```python
from build123d import *

# Parameters (mm, degrees)
BOSS_EXTRUDE1_DEPTH     = 5
SKETCH2_W               = 30
SKETCH2_H               = 15
BOSS_EXTRUDE2_DEPTH     = 25
CUT_EXTRUDE1_DEPTH      = 44.373378932
SKETCH3_3_R             = 14
SKETCH3_3_R_2           = 13
CUT_EXTRUDE2_DEPTH      = 1
CUT_EXTRUDE3_DEPTH      = 44.373378932
CUT_EXTRUDE3_DEPTH_BACK = 44.373378932
SKETCH3_4_R             = 4
SKETCH3_5_R             = 13
SKETCH3_5_R_2           = 5
CUT_EXTRUDE4_DEPTH      = 3
CUT_EXTRUDE5_START      = 3
SKETCH5_R               = 13
SKETCH5_R_2             = 5
CUT_EXTRUDE5_DEPTH      = 3
CUT_EXTRUDE8_START      = 1
SKETCH5_8_R             = 14
SKETCH5_8_R_2           = 13
CUT_EXTRUDE8_DEPTH      = 1
CUT_EXTRUDE9_START      = 2
SKETCH5_9_R             = 5
SKETCH5_9_R_2           = 4
CUT_EXTRUDE9_DEPTH      = 2
SKETCH6_R               = 2.65
CUT_EXTRUDE10_DEPTH     = 38.91437722


with BuildPart() as part:
    # Sketch1 → Boss-Extrude1 (new body)
    with BuildSketch(Plane(origin=(0, 0, 0), x_dir=(1, 0, 0), z_dir=(0, 1, 0))):
        Polygon((25.5, 7.5), (27.5, 5.5), (27.5, -5.5), (25.5, -7.5), (-25.5, -7.5), (-27.5, -5.5), (-27.5, 5.5), (-25.5, 7.5), align=None)
    extrude(amount=BOSS_EXTRUDE1_DEPTH)

    # Sketch2 → Boss-Extrude2 (add)
    with BuildSketch(Plane(origin=(0, 5, 0), x_dir=(1, 0, 0), z_dir=(0, 1, 0))):
        Rectangle(SKETCH2_W, SKETCH2_H)
    extrude(amount=BOSS_EXTRUDE2_DEPTH)

    # Sketch3 → Cut-Extrude1 (cut, through all)
    with BuildSketch(Plane.XY.offset(7.5)):
        with BuildLine():
            Line((-15, 30), (-15, 15.652790041))
            ThreePointArc((-15, 15.652790041), (-10.616641061, 25.616641061), (-0.652790041, 30))
            Line((-0.652790041, 30), (-15, 30))
        make_face()
        with BuildLine():
            ThreePointArc((0.652790041, 30), (10.616641061, 25.616641061), (15, 15.652790041))
            Line((15, 15.652790041), (15, 30))
            Line((15, 30), (0.652790041, 30))
        make_face()
    extrude(amount=-CUT_EXTRUDE1_DEPTH, mode=Mode.SUBTRACT)

    # Sketch3<3> → Cut-Extrude2 (cut)
    with BuildSketch(Plane.XY.offset(7.5)):
        with Locations((0, 15)):
            Circle(SKETCH3_3_R)
        with Locations((0, 15)):
            Circle(SKETCH3_3_R_2, mode=Mode.SUBTRACT)
    extrude(amount=-CUT_EXTRUDE2_DEPTH, mode=Mode.SUBTRACT)

    # Sketch3<4> → Cut-Extrude3 (cut, two sides: drawn at the far end of the back side and taken through both)
    with BuildSketch(Plane.XY.offset(7.5).offset(-CUT_EXTRUDE3_DEPTH_BACK)):
        with Locations((0, 15)):
            Circle(SKETCH3_4_R)
    extrude(amount=CUT_EXTRUDE3_DEPTH + CUT_EXTRUDE3_DEPTH_BACK, mode=Mode.SUBTRACT)

    # Sketch3<5> → Cut-Extrude4 (cut)
    with BuildSketch(Plane.XY.offset(7.5)):
        with Locations((0, 15)):
            Circle(SKETCH3_5_R)
        with Locations((0, 15)):
            Circle(SKETCH3_5_R_2, mode=Mode.SUBTRACT)
    extrude(amount=-CUT_EXTRUDE4_DEPTH, mode=Mode.SUBTRACT)

    # Sketch5 → Cut-Extrude5 (cut)
    with BuildSketch(Plane.XY.offset(-7.5).offset(CUT_EXTRUDE5_START)):
        with Locations((0, 15)):
            Circle(SKETCH5_R)
        with Locations((0, 15)):
            Circle(SKETCH5_R_2, mode=Mode.SUBTRACT)
    extrude(amount=-CUT_EXTRUDE5_DEPTH, mode=Mode.SUBTRACT)

    # Sketch5<8> → Cut-Extrude8 (cut)
    with BuildSketch(Plane.XY.offset(-7.5).offset(CUT_EXTRUDE8_START)):
        with Locations((0, 15)):
            Circle(SKETCH5_8_R)
        with Locations(Location((0, 15, 0), (0, 0, 180))):
            Circle(SKETCH5_8_R_2, mode=Mode.SUBTRACT)
    extrude(amount=-CUT_EXTRUDE8_DEPTH, mode=Mode.SUBTRACT)

    # Sketch5<9> → Cut-Extrude9 (cut)
    with BuildSketch(Plane.XY.offset(-7.5).offset(CUT_EXTRUDE9_START)):
        with Locations(Location((0, 15, 0), (0, 0, 180))):
            Circle(SKETCH5_9_R)
        with Locations((0, 15)):
            Circle(SKETCH5_9_R_2, mode=Mode.SUBTRACT)
    extrude(amount=-CUT_EXTRUDE9_DEPTH, mode=Mode.SUBTRACT)

    # Sketch6 → Cut-Extrude10 (cut, through all)
    with BuildSketch(Plane(origin=(0, 5, 0), x_dir=(1, 0, 0), z_dir=(0, 1, 0))):
        with Locations(Location((-21.25, 0, 0), (0, 0, 270))):
            Circle(SKETCH6_R)
        with Locations(Location((21.25, 0, 0), (0, 0, 270))):
            Circle(SKETCH6_R)
    extrude(amount=-CUT_EXTRUDE10_DEPTH, mode=Mode.SUBTRACT)


solid = part.part
```
The listing builds one solid part. Answer for the finished solid, in the listing's coordinates (mm). A direction names the side the tool comes from. Coordinates: 2 decimals unless noted, no trailing zeros. Order: outer loops, then holes, each group sorted by start corner. A loop starts at its lowest first (then second) coordinate and runs counter-clockwise, first axis right, second up. Notation, with made-up numbers: M 21.25,42 L 67.25,42 A18 cw 67.25,48 Z; hole C 84.25,-9.5 d7. An arc over 180 degrees is marked long. Answer as a JSON object with one key per item and string values. Group by question number.
1. Determine the mould class of faces 1 (the flat face through (0, 0, 0)), 2 (the flat face through (6, 15, 4.5)), 3 (the flat face through (26, 2, -7)) for opening direction Y: released by +Y, released by -Y, zero draft, split by the parting line, or undercut.
2. A tool of negligible diameter and unlimited length cuts with its end or side. For faces 4 (the flat face through (15, 10, 0)), 5 (the cylindrical face through (-9.58, 23.79, -5.49)), 6 (the flat face through (9.3, 5.7, 6.5)), from which of +Z, -Z, +X, -X, +Y, -Y can it reach the whole face along a straight path? Write none if from no direction.
3. Section D-D on y = 22.5 is taken. Write down the section's boundary in (x, z), then the cut area to 3 significant figures.
4. Straight lines are drawn through the part: line 1 (X direction, y = 1.1, z = 0); line 2 (Y direction, x = 0, z = 5.55); line 3 (Y direction, x = 0, z = -6.8). For each, find the intervals that lie inside material, in ascending order.
5. Section A-A on z = 0 is taken. Write down the section's boundary in (x, y).
6. Section B-B on x = 21.25 is taken. Write down the section's boundary in (y, z), then the cut area to 3 significant figures.
7. Flat-ended cylindrical pins translate along their axes: P1, Ø6, axis at x = -23.5, z = 0, coming from the +Y side; P2, Ø6, axis at y = 18.5, z = -0.5, coming from the +X side; P3, Ø8, axis at x = -2.5, y = 17, coming from the -Z side. Find the tip coordinate at first contact, or state that the pin passes through.
Values follow:
{
 "1": {"face 1": "released by -Y", "face 2": "undercut", "face 3": "zero draft"},
 "2": {"face 4": "+Z, -Z, +X, +Y", "face 5": "-Z", "face 6": "+Z"},
 "3": {"outline": "M -13.01,-7.5 L -11.82,-7.5 L -11.82,-6.5 L -10.62,-6.5 L -10.62,-4.5 L 10.62,-4.5 L 10.62,-6.5 L 11.82,-6.5 L 11.82,-7.5 L 13.01,-7.5 L 13.01,7.5 L 11.82,7.5 L 11.82,6.5 L 10.62,6.5 L 10.62,4.5 L -10.62,4.5 L -10.62,6.5 L -11.82,6.5 L -11.82,7.5 L -13.01,7.5 Z", "area": "258 mm2"},
 "4": {"line 1": "-27.5 to -23.9, -18.6 to 18.6, 23.9 to 27.5", "line 2": "0 to 2, 10 to 11, 19 to 20, 28 to 30", "line 3": "0 to 1, 29 to 30"},
 "5": {"outline": "M -27.5,0 L -23.9,0 L -23.9,5 L -27.5,5 Z; M -18.6,0 L 18.6,0 L 18.6,5 L 15,5 L 15,15.65 A15.01 ccw 0.65,30 L -0.65,30 A15.01 ccw -15,15.65 L -15,5 L -18.6,5 Z; M 23.9,0 L 27.5,0 L 27.5,5 L 23.9,5 Z; hole C 0,15 d8"},
 "6": {"outline": "M 0,-7.5 L 5,-7.5 L 5,-2.65 L 0,-2.65 Z; M 0,2.65 L 5,2.65 L 5,7.5 L 0,7.5 Z", "area": "48.5 mm2"},
 "7": {"P1": "y = 5", "P2": "x = 15", "P3": "z = -5.5"}
}
